from build123d import *

# Parameters (mm, degrees)
SALIENTE_EXTRUIR1_DEPTH = 1
CROQUIS3_W              = 100
CROQUIS3_H              = 40
SALIENTE_EXTRUIR2_DEPTH = 1
CROQUIS5_W              = 10.5
CROQUIS5_H              = 8.1
SALIENTE_EXTRUIR3_DEPTH = 20
SALIENTE_EXTRUIR4_DEPTH = 20
CROQUIS7_R              = 3.25
CORTAR_EXTRUIR1_DEPTH   = 100
REDONDEO2_R             = 5
CHAFL_N2_SIZE           = 1
REDONDEO3_R             = 1
REDONDEO4_R             = 0.5
REDONDEO5_R             = 0.5


with BuildPart() as part:
    # Croquis1 → Saliente-Extruir1 (new body)
    with BuildSketch(Plane.XY.offset(20)):
        Polygon((-50, 0), (50, 0), (0, 28.867513459), align=None)
    extrude(amount=-SALIENTE_EXTRUIR1_DEPTH)


with BuildPart() as body_2:
    # Simetría4: mirrored copy
    add(part.part.mirror(Plane.XY))


with BuildPart() as part_1:
    add(part.part)

    add(body_2.part)  # Saliente-Extruir2 merges body 2
    # Croquis3 → Saliente-Extruir2 (add)
    with BuildSketch(Plane(origin=(0, 0, 0), x_dir=(1, 0, 0), z_dir=(0, 1, 0))):
        Rectangle(CROQUIS3_W, CROQUIS3_H)
    extrude(amount=-SALIENTE_EXTRUIR2_DEPTH)

    # Croquis5 → Saliente-Extruir3 (add, symmetric)
    with BuildSketch(Plane.XY):
        with Locations((0, -5.05)):
            Rectangle(CROQUIS5_W, CROQUIS5_H)
    extrude(amount=SALIENTE_EXTRUIR3_DEPTH, both=True)

    # Croquis6 → Saliente-Extruir4 (add, symmetric)
    with BuildSketch(Plane.XY):
        Polygon((0, 28.867513459), (9.379623704, 0), (-9.379623704, 0), align=None)
    extrude(amount=SALIENTE_EXTRUIR4_DEPTH, both=True)

    # Croquis7 → Cortar-Extruir1 (cut, symmetric)
    with BuildSketch(Plane.XY.offset(-19)):
        with Locations(Location((0, -3.85, 0), (0, 0, 180))):
            Circle(CROQUIS7_R)
    extrude(amount=CORTAR_EXTRUIR1_DEPTH, both=True, mode=Mode.SUBTRACT)

    # Redondeo2
    redondeo2_edges = [part_1.edges().sort_by_distance(p)[0] for p in [
        (-5.25, -9.1, 0),
        (5.25, -9.1, 0),
    ]]
    fillet(redondeo2_edges, radius=REDONDEO2_R)

    # Chaflán2
    chafl_n2_edges = [part_1.edges().sort_by_distance(p)[0] for p in [
        (3.25, -3.85, -20),
        (3.25, -3.85, 20),
    ]]
    chamfer(chafl_n2_edges, length=CHAFL_N2_SIZE)

    # Redondeo3
    redondeo3_edges = [part_1.edges().sort_by_distance(p)[0] for p in [
        (5.25, -1, 0),
        (-5.25, -1, 0),
    ]]
    fillet(redondeo3_edges, radius=REDONDEO3_R)

    # Redondeo4
    redondeo4_edges = [part_1.edges().sort_by_distance(p)[0] for p in [
        (-5.542893219, -1.292893219, 20),
        (-28.125, -1, 20),
        (28.125, -1, -20),
        (5.25, -3.05, -20),
        (5.25, -3.05, 20),
        (0, -9.1, -20),
        (-3.785533906, -7.635533906, -20),
        (3.785533906, -7.635533906, -20),
        (0, -9.1, 20),
        (-3.785533906, -7.635533906, 20),
        (3.785533906, -7.635533906, 20),
        (28.125, -1, 20),
        (-5.25, -3.05, -20),
        (-5.25, -3.05, 20),
        (-28.125, -1, -20),
        (5.542893219, -1.292893219, -20),
        (5.542893219, -1.292893219, 20),
        (-5.542893219, -1.292893219, -20),
    ]]
    fillet(redondeo4_edges, radius=REDONDEO4_R)

    # Redondeo5
    # the kernel refuses this fillet: 0.5 mm, written as the material it takes off along each edge
    with BuildSketch(Plane(origin=(1.082531755, 29.492513459, 19), x_dir=(0, 0, 1), z_dir=(-0.8660254037844387, -0.5000000000000001, 0))) as redondeo5_piece_1_section:
        with BuildLine():
            CenterArc((REDONDEO5_R, -REDONDEO5_R), REDONDEO5_R, 90, 90)
            Line((0, -REDONDEO5_R), (0, 0))
            Line((0, 0), (REDONDEO5_R, 0))
        make_face()
    redondeo5_piece_1 = extrude(amount=60.235026919, mode=Mode.PRIVATE)
    redondeo5_piece_1 = split(redondeo5_piece_1, bisect_by=Plane(origin=(0.055315574, 28.697269627, 19.065385241), z_dir=(0.9510565162951544, 0.30901699437494506, 0)), keep=Keep.TOP, mode=Mode.PRIVATE)
    add(redondeo5_piece_1, mode=Mode.SUBTRACT)
    with BuildSketch(Plane(origin=(1.082531755, 29.492513459, 19), x_dir=(0, 0, 1), z_dir=(-0.8660254037844387, -0.5000000000000001, 0))) as redondeo5_piece_2_section:
        with BuildLine():
            CenterArc((REDONDEO5_R, -REDONDEO5_R), REDONDEO5_R, 90, 90)
            Line((0, -REDONDEO5_R), (0, 0))
            Line((0, 0), (REDONDEO5_R, 0))
        make_face()
    redondeo5_piece_2 = extrude(amount=60.235026919, mode=Mode.PRIVATE)
    redondeo5_piece_2 = split(redondeo5_piece_2, bisect_by=Plane(origin=(-24.914439582, 0, 19.11193997), z_dir=(0, 1, 0)), keep=Keep.TOP, mode=Mode.PRIVATE)
    redondeo5_piece_2 = split(redondeo5_piece_2, bisect_by=Plane(origin=(-6.644327312, 8.418376676, 19.11193997), z_dir=(-0.9510565162951545, 0.30901699437494473, 0)), keep=Keep.TOP, mode=Mode.PRIVATE)
    add(redondeo5_piece_2, mode=Mode.SUBTRACT)
    with BuildSketch(Plane(origin=(51.082531755, -0.625, -19), x_dir=(0, 0, -1), z_dir=(-0.8660254037844388, 0.49999999999999983, 0))) as redondeo5_piece_3_section:
        with BuildLine():
            CenterArc((REDONDEO5_R, REDONDEO5_R), REDONDEO5_R, 180, 90)
            Line((0, REDONDEO5_R), (0, 0))
            Line((0, 0), (REDONDEO5_R, 0))
        make_face()
    redondeo5_piece_3 = extrude(amount=60.235026919, mode=Mode.PRIVATE)
    redondeo5_piece_3 = split(redondeo5_piece_3, bisect_by=Plane(origin=(24.914439582, 0, -19.11193997), z_dir=(0, 1, 0)), keep=Keep.TOP, mode=Mode.PRIVATE)
    redondeo5_piece_3 = split(redondeo5_piece_3, bisect_by=Plane(origin=(6.644327312, 8.418376676, -19.11193997), z_dir=(0.9510565162951544, 0.30901699437494506, 0)), keep=Keep.TOP, mode=Mode.PRIVATE)
    add(redondeo5_piece_3, mode=Mode.SUBTRACT)
    with BuildSketch(Plane(origin=(51.082531755, -0.625, -19), x_dir=(0, 0, -1), z_dir=(-0.8660254037844388, 0.49999999999999983, 0))) as redondeo5_piece_4_section:
        with BuildLine():
            CenterArc((REDONDEO5_R, REDONDEO5_R), REDONDEO5_R, 180, 90)
            Line((0, REDONDEO5_R), (0, 0))
            Line((0, 0), (REDONDEO5_R, 0))
        make_face()
    redondeo5_piece_4 = extrude(amount=60.235026919, mode=Mode.PRIVATE)
    redondeo5_piece_4 = split(redondeo5_piece_4, bisect_by=Plane(origin=(-0.055315574, 28.697269627, -19.065385241), z_dir=(-0.9510565162951545, 0.30901699437494473, 0)), keep=Keep.TOP, mode=Mode.PRIVATE)
    add(redondeo5_piece_4, mode=Mode.SUBTRACT)
    with BuildSketch(Plane(origin=(1.082531755, 29.492513459, -19), x_dir=(0, 0, -1), z_dir=(-0.8660254037844387, -0.5000000000000001, 0))) as redondeo5_piece_5_section:
        with BuildLine():
            CenterArc((REDONDEO5_R, REDONDEO5_R), REDONDEO5_R, 180, 90)
            Line((0, REDONDEO5_R), (0, 0))
            Line((0, 0), (REDONDEO5_R, 0))
        make_face()
    redondeo5_piece_5 = extrude(amount=60.235026919, mode=Mode.PRIVATE)
    redondeo5_piece_5 = split(redondeo5_piece_5, bisect_by=Plane(origin=(0.055315574, 28.697269627, -19.065385241), z_dir=(0.9510565162951544, 0.30901699437494506, 0)), keep=Keep.TOP, mode=Mode.PRIVATE)
    add(redondeo5_piece_5, mode=Mode.SUBTRACT)
    with BuildSketch(Plane(origin=(1.082531755, 29.492513459, -19), x_dir=(0, 0, -1), z_dir=(-0.8660254037844387, -0.5000000000000001, 0))) as redondeo5_piece_6_section:
        with BuildLine():
            CenterArc((REDONDEO5_R, REDONDEO5_R), REDONDEO5_R, 180, 90)
            Line((0, REDONDEO5_R), (0, 0))
            Line((0, 0), (REDONDEO5_R, 0))
        make_face()
    redondeo5_piece_6 = extrude(amount=60.235026919, mode=Mode.PRIVATE)
    redondeo5_piece_6 = split(redondeo5_piece_6, bisect_by=Plane(origin=(-24.914439582, 0, -19.11193997), z_dir=(0, 1, 0)), keep=Keep.TOP, mode=Mode.PRIVATE)
    redondeo5_piece_6 = split(redondeo5_piece_6, bisect_by=Plane(origin=(-6.644327312, 8.418376676, -19.11193997), z_dir=(-0.9510565162951545, 0.30901699437494473, 0)), keep=Keep.TOP, mode=Mode.PRIVATE)
    add(redondeo5_piece_6, mode=Mode.SUBTRACT)
    with BuildSketch(Plane(origin=(51.082531755, -0.625, 19), x_dir=(0, 0, 1), z_dir=(-0.8660254037844388, 0.49999999999999983, 0))) as redondeo5_piece_7_section:
        with BuildLine():
            CenterArc((REDONDEO5_R, -REDONDEO5_R), REDONDEO5_R, 90, 90)
            Line((0, -REDONDEO5_R), (0, 0))
            Line((0, 0), (REDONDEO5_R, 0))
        make_face()
    redondeo5_piece_7 = extrude(amount=60.235026919, mode=Mode.PRIVATE)
    redondeo5_piece_7 = split(redondeo5_piece_7, bisect_by=Plane(origin=(24.914439582, 0, 19.11193997), z_dir=(0, 1, 0)), keep=Keep.TOP, mode=Mode.PRIVATE)
    redondeo5_piece_7 = split(redondeo5_piece_7, bisect_by=Plane(origin=(6.644327312, 8.418376676, 19.11193997), z_dir=(0.9510565162951544, 0.30901699437494506, 0)), keep=Keep.TOP, mode=Mode.PRIVATE)
    add(redondeo5_piece_7, mode=Mode.SUBTRACT)
    with BuildSketch(Plane(origin=(51.082531755, -0.625, 19), x_dir=(0, 0, 1), z_dir=(-0.8660254037844388, 0.49999999999999983, 0))) as redondeo5_piece_8_section:
        with BuildLine():
            CenterArc((REDONDEO5_R, -REDONDEO5_R), REDONDEO5_R, 90, 90)
            Line((0, -REDONDEO5_R), (0, 0))
            Line((0, 0), (REDONDEO5_R, 0))
        make_face()
    redondeo5_piece_8 = extrude(amount=60.235026919, mode=Mode.PRIVATE)
    redondeo5_piece_8 = split(redondeo5_piece_8, bisect_by=Plane(origin=(-0.055315574, 28.697269627, 19.065385241), z_dir=(-0.9510565162951545, 0.30901699437494473, 0)), keep=Keep.TOP, mode=Mode.PRIVATE)
    add(redondeo5_piece_8, mode=Mode.SUBTRACT)


solid = part_1.part
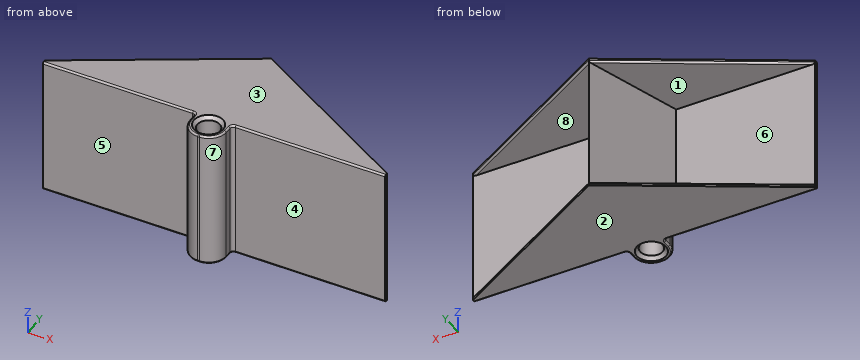
For this review, take the finished solid that the model builds, in its own axes (mm). Face numbers are marked on the shaded views. A direction names the side the tool comes from. Round coordinates to 2 decimals unless told otherwise and drop trailing zeros. Order: outer loops, then holes, each group sorted by start corner. A loop starts at its lowest first (then second) coordinate and runs counter-clockwise, first axis right, second up. Notation, with made-up numbers: M -27.75,49.5 L 7.25,49.5 A19 cw 7.25,64.5 Z; hole C 38,45 d10. An arc over 180 degrees is marked long. Use a Markdown table: item, result. Add a question column.
Item 1: Insertion check: pin 1 (3 mm diameter, centred on x = -16, z = 2, fed in from -Y); pin 2 (0.6 mm diameter, centred on y = -2.5, z = 3, fed in from +X); pin 3 (4 mm diameter, centred on y = 19.5, z = -0.5, fed in from +X). Each pin has a flat end and moves straight along its axis. Give the tip position at first contact, or say it passes through.
Item 2: Mouldability with a two-part tool opening along Z and no side actions: class the marked faces 1, 2, 3 and 4 as released by +Z, released by -Z, zero draft, split by the parting line, or undercut.
Item 3: To check wall thickness, follow line 1 along Z through (x, y) = (-15.5, 8.5); line 2 along Y through (x, z) = (-27, 16.5); line 3 along X through (y, z) = (24, -11.5). State the ranges of each line that lie inside material, in increasing order.
Item 4: Tool access review of the marked faces 5, 6, 7 and 8: name each direction out of +Z, -Z, +X, -X, +Y, -Y from which nothing blocks a thin tool from reaching the whole face with its end or side.
Item 5: Add section A-A, the plane z = -1. Give the boundary of the cut face in (x, y).
Geometry results:
| question | item | result |
|---|---|---|
| 1 | pin 1 | stops at y = -1 |
| 1 | pin 2 | stops at x = 5.25 |
| 1 | pin 3 | stops at x = 3.69 |
| 2 | face 1 | undercut |
| 2 | face 2 | released by -Z |
| 2 | face 3 | released by +Z |
| 2 | face 4 | zero draft |
| 3 | line 1 | z = -20 to -19, 19 to 20 |
| 3 | line 2 | y = -1 to 0 |
| 3 | line 3 | x = -1.58 to 1.58 |
| 4 | face 5 | +Z, -Z, -X, -Y |
| 4 | face 6 | -X, +Y |
| 4 | face 7 | +Z, -Z, +X, -Y |
| 4 | face 8 | +X, +Y |
| 5 | outline | M -50,-1 L -6.25,-1 A1 cw -5.25,-2 L -5.25,-4.1 A5 ccw -0.25,-9.1 L 0.25,-9.1 A5 ccw 5.25,-4.1 L 5.25,-2 A1 cw 6.25,-1 L 50,-1 L 50,0 L 9.38,0 L 0,28.87 L -9.38,0 L -50,0 Z; hole C 0,-3.85 d6.5 |
